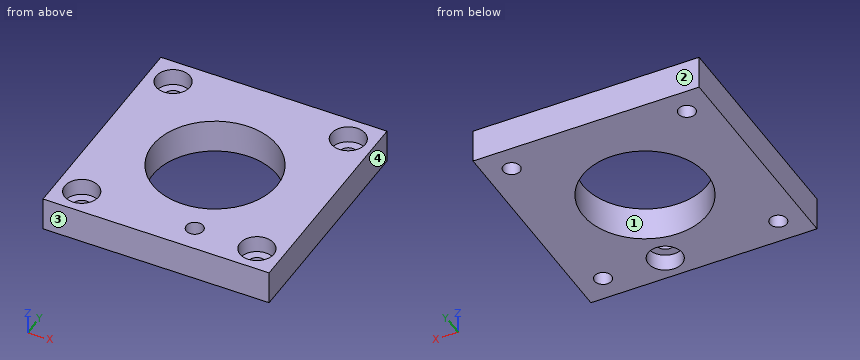
```python
from build123d import *

# Parameters (mm, degrees)
F0_R           = 11
F1_DEPTH       = 6
F2_D           = 3
F2_CBORE_D     = 6
F2_CBORE_DEPTH = 3
F4_D           = 3
F4_CBORE_D     = 6
F4_CBORE_DEPTH = 3


with BuildPart() as f1:
    # F0 (on Top) → F1 (new body)
    with BuildSketch(Plane.XY):
        Polygon((0, -20), (20, -20), (20, 20), (-20, 20), (-20, -20), align=None)
        Polygon((15.5, -15.5), (0, -15.5), (-15.5, -15.5), (-15.5, 15.5), (15.5, 15.5), align=None, mode=Mode.SUBTRACT)
        Polygon((-15.5, -15.5), (0, -15.5), (15.5, -15.5), (15.5, 15.5), (-15.5, 15.5), align=None)
        Circle(F0_R, mode=Mode.SUBTRACT)
    extrude(amount=-F1_DEPTH)

    # F2 (through all)
    with Locations(Plane.XY):
        with Locations((15.5, 15.5), (15.5, -15.5), (-15.5, -15.5), (-15.5, 15.5)):
            CounterBoreHole(F2_D / 2, F2_CBORE_D / 2, F2_CBORE_DEPTH)

    # F4 (through all)
    with Locations(Plane(origin=(0, 0, -6), x_dir=(1, 0, 0), z_dir=(0, 0, -1))):
        with Locations((4.5, 15.5)):
            CounterBoreHole(F4_D / 2, F4_CBORE_D / 2, F4_CBORE_DEPTH)


solid = f1.part
```
Could you check a few things on this model? Use its own coordinates, in mm. Face numbers are marked on the shaded views. Round coordinates to 2 decimals unless told otherwise and drop trailing zeros. Write each loop counter-clockwise with the first axis right and the second up, starting at its lowest first coordinate (ties: lowest second). Pieces come first, ordered by that corner, then holes.
(1) For pin 1 (3 mm diameter, centred on x = -14.5, y = -15, fed in from +Z), with a flat end and sliding along its axis, tell me the tip position at first contact or that it passes through.
Findings below:
pin 1: stops at z = -3
(2) Suppose I cut it at B-B on x = 0. Write out the boundary of the cut face in (y, z), and give its area (3 significant figures).
Findings below:
outline: (-20, -6) - (-11, -6) - (-11, 0) - (-20, 0) - close; (11, -6) - (20, -6) - (20, 0) - (11, 0) - close
area: 108 mm2
(3) Suppose I cut it at A-A on y = 15.5. Write out the boundary of the cut face in (x, z).
Findings below:
outline: (-20, -6) - (-17, -6) - (-17, -3) - (-18.5, -3) - (-18.5, 0) - (-20, 0) - close; (-14, -6) - (14, -6) - (14, -3) - (12.5, -3) - (12.5, 0) - (-12.5, 0) - (-12.5, -3) - (-14, -3) - close; (17, -6) - (20, -6) - (20, 0) - (18.5, 0) - (18.5, -3) - (17, -3) - close
(4) Thinking about a two-plate mould opening in Y: for the marked faces 1, 2, 3 and 4, which applies, +Y half, -Y half, draft (parallel to the pull), parting line (faces both ways), or undercut?
Findings below:
face 1: undercut
face 2: +Y half
face 3: -Y half
face 4: draft
(5) If I drill on probe 1 along Y at (x, z) = (15.5, -1.15); probe 2 along Y at (x, z) = (5, -5.6); probe 3 along Y at (x, z) = (-0.5, -5.6), over which ranges is the centre line in solid material (lowest first)?
Findings below:
probe 1: y = -20 to -18.5, -12.5 to 12.5, 18.5 to 20
probe 2: y = -20 to -18.46, -12.54 to -9.8, 9.8 to 20
probe 3: y = -20 to -10.99, 10.99 to 20
(6) Suppose I cut it at D-D on z = -1.7. Write out the boundary of the cut face in (x, y).
Findings below:
outline: (-20, -20) - (20, -20) - (20, 20) - (-20, 20) - close; hole circle Ø6 at (-15.5, -15.5); hole circle Ø6 at (-15.5, 15.5); hole circle Ø22 at (0, 0); hole circle Ø3 at (4.5, -15.5); hole circle Ø6 at (15.5, -15.5); hole circle Ø6 at (15.5, 15.5)
